```python
from build123d import *

# Parameters (mm, degrees)
EXTRUDE_DEPTH   = 3.3
SKETCH001_R     = 1.5
POCKET_DEPTH    = 3.301
SKETCH002_R     = 3
POCKET001_DEPTH = 5


with BuildPart() as part:
    # Sketch → Extrude (new body)
    with BuildSketch(Plane.XY):
        with BuildLine():
            ThreePointArc((3.5, 21.5), (0, 25), (-3.5, 21.5))
            Line((-3.5, 21.5), (-3.5, 19.691369))
            ThreePointArc((-3.5, 19.691369), (0, -20), (3.5, 19.691369))
            Line((3.5, 19.691369), (3.5, 21.5))
        make_face()
    extrude(amount=EXTRUDE_DEPTH)

    # Sketch001 (on Face6 of Extrude) → Pocket (cut, through all)
    with BuildSketch(Plane.XY.offset(3.3)):
        with Locations((0, 21.5)):
            Circle(SKETCH001_R)
    extrude(amount=-POCKET_DEPTH, mode=Mode.SUBTRACT)

    # Sketch002 → Pocket001 (cut)
    with BuildSketch(Plane.XY.offset(3.3)):
        with Locations((-9, 9)):
            Circle(SKETCH002_R)
        with Locations((9, 9)):
            Circle(SKETCH002_R)
        with BuildLine():
            Line((-13, -7.483315), (13, -7.483315))
            ThreePointArc((-13, -7.483315), (0, -15), (13, -7.483315))
        make_face()
    extrude(amount=-POCKET001_DEPTH, mode=Mode.SUBTRACT)


solid = part.part
```
Geometry: final body of the model. Coordinates: model frame, mm. A direction names the side the tool comes from. Round coordinates to 2 decimals unless told otherwise and drop trailing zeros. Order: outer loops, then holes, each group sorted by start corner. A loop starts at its lowest first (then second) coordinate and runs counter-clockwise, first axis right, second up. Notation, with made-up numbers: (4.25, 53) - (23.25, 53) arc R24 cw to (23.25, 70) - close; hole circle Ø4 at (48.25, 10.5). An arc over 180 degrees is marked (long way). Use CSV: the item, a comma, the result in double quotes. Start each with the question number.
Q1. Section query B-B (y = 11). Return loops of the section in (x, z), and give its area (3 significant figures).
Q2. Section query D-D (y = -12.5). Return loops of the section in (x, z), and give its area (3 significant figures).
Q3. First-contact query: pin 1 (7 mm diameter, centred on x = 9, y = 9, fed in from +Z); pin 2 (1 mm diameter, centred on x = 4.5, z = 1, fed in from +Y); pin 3 (1.5 mm diameter, centred on y = 5, z = 2, fed in from +X). Flat tips, straight axial feed; report the tip coordinate or a pass-through.
Q4. Section query A-A (x = 0). Return loops of the section in (y, z), and give its area (3 significant figures).
Q5. Material intervals for line 1 along Y through (x, z) = (-8, 1.7); line 2 along Y through (x, z) = (-0.5, 2.8); line 3 along X through (y, z) = (-11, 3.15), sorted ascending. Write a range as from..to.
Q6. Access query for faces 1 (the face through (0, -7.483, 2)), 2 (the face through (-3.5, 21, 2)), 3 (the face through (0, 3, 3.3)), 4 (the face through (3.5, 21, 2)). Directions: +Z, -Z, +X, -X, +Y, -Y. A direction counts if a zero-diameter tool reaches every point of the face in a straight line with its end or side. Return the directions, or none.
Q7. Section query C-C (z = 2.15). Return loops of the section in (x, y), and give its area (3 significant figures).
Result set:
1,outline,"(-16.7, 0) - (-11.24, 0) - (-11.24, 3.3) - (-16.7, 3.3) - close; (-6.76, 0) - (6.76, 0) - (6.76, 3.3) - (-6.76, 3.3) - close; (11.24, 0) - (16.7, 0) - (16.7, 3.3) - (11.24, 3.3) - close"
1,area,"80.7 mm2"
2,outline,"(-15.61, 0) - (-8.29, 0) - (-8.29, 3.3) - (-15.61, 3.3) - close; (8.29, 0) - (15.61, 0) - (15.61, 3.3) - (8.29, 3.3) - close"
2,area,"48.3 mm2"
3,pin 1,"stops at z = 3.3"
3,pin 2,"stops at y = 19.6"
3,pin 3,"stops at x = 19.54"
4,outline,"(-20, 0) - (-15, 0) - (-15, 3.3) - (-20, 3.3) - close; (-7.48, 0) - (20, 0) - (20, 3.3) - (-7.48, 3.3) - close; (23, 0) - (25, 0) - (25, 3.3) - (23, 3.3) - close"
4,area,"114 mm2"
5,line 1,"y = -18.33..-12.69, -7.48..6.17, 11.83..18.33"
5,line 2,"y = -19.99..-14.99, -7.48..20.09, 22.91..24.96"
5,line 3,"x = -16.7..-10.2, 10.2..16.7"
6,face 1,"+Z, -Z"
6,face 2,"+Z, -Z, -X, +Y"
6,face 3,"+Z, +X, -X, +Y, -Y"
6,face 4,"+Z, -Z, +X, +Y"
7,outline,"(-3.5, 19.69) arc R20 ccw (long way) to (3.5, 19.69) - (3.5, 21.5) arc R3.5 ccw to (-3.5, 21.5) - close; hole (-13, -7.48) arc R15 ccw to (13, -7.48) - close; hole circle Ø6 at (-9, 9); hole circle Ø3 at (0, 21.5); hole circle Ø6 at (9, 9)"
7,area,"1,080 mm2"
